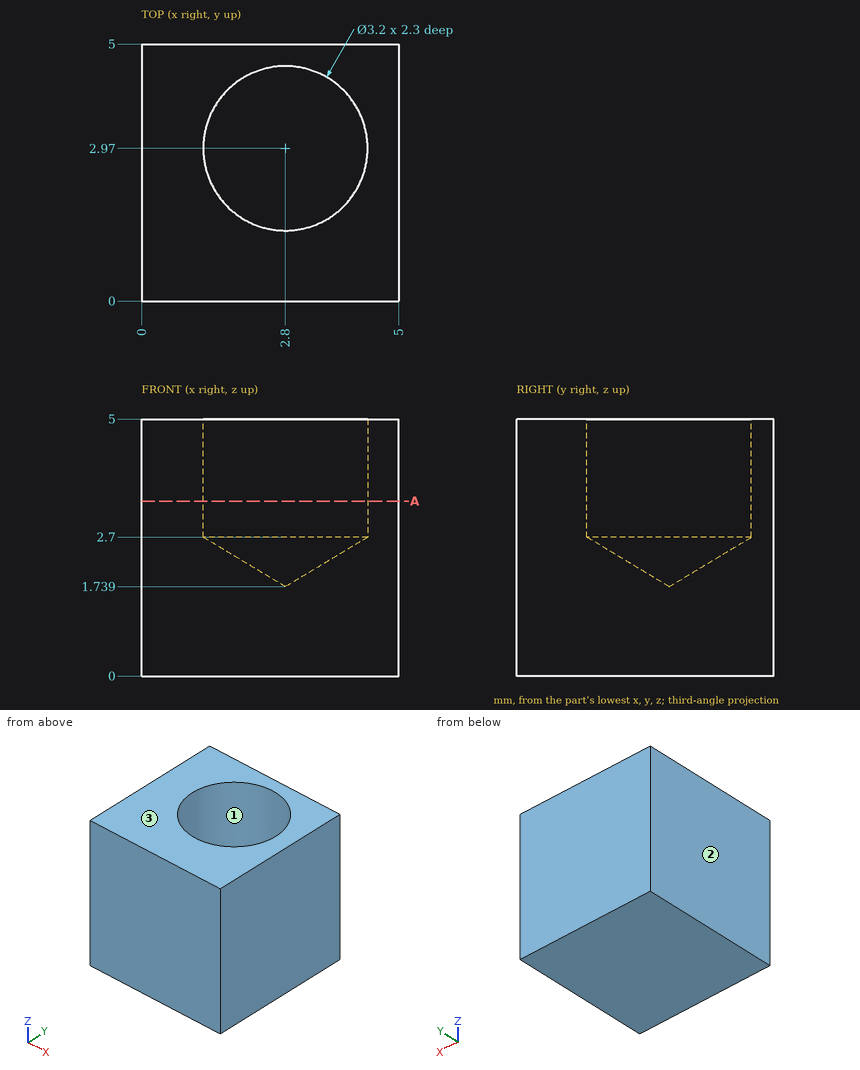
Here's the drawing with two shaded views (mm, measured from the low corner). I have some questions. Coordinates: 2 decimals unless noted, no trailing zeros. Loops run counter-clockwise (first coordinate to the right, second up) from the corner with the lowest first, then second, coordinate; pieces in that order, holes last. Notation, with made-up numbers: M 83,48.5 L 100,48.5 A26 ccw 100,81.5 Z; hole C 12.25,61 d7. An arc over 180 degrees is marked long. Put each result on its own line as item: value. Start each with the question number.
(1) I need wall thicknesses on probe 1 along Y at (x, z) = (2.8, 3.8); probe 2 along X at (y, z) = (2.25, 3.3); probe 3 along Y at (x, z) = (1.7, 3.85). Which ranges of each line are inside material? Lowest first, please.
(2) Imagine slicing it at A-A on z = 3.4. List the corners of the cut face in (x, y) for me.
(3) We'd pull the mould along X, two halves only. Please class the marked faces 1, 2 and 3: +X half, -X half, draft (parallel to the pull), parting line (faces both ways), or undercut.
(4) Will this pin go through, and if not, where does the flat tip stop? pin 1 Ø3 at (x, y) = (4.5, 3) entering from -Z.
Worked answers:
1. probe 1: y = 0 to 1.37, 4.57 to 5
1. probe 2: x = 0 to 1.37, 4.23 to 5
1. probe 3: y = 0 to 1.81, 4.13 to 5
2. outline: M 0,0 L 5,0 L 5,5 L 0,5 Z; hole C 2.8,2.97 d3.2
3. face 1: undercut
3. face 2: -X half
3. face 3: draft
4. pin 1: stops at z = 0
